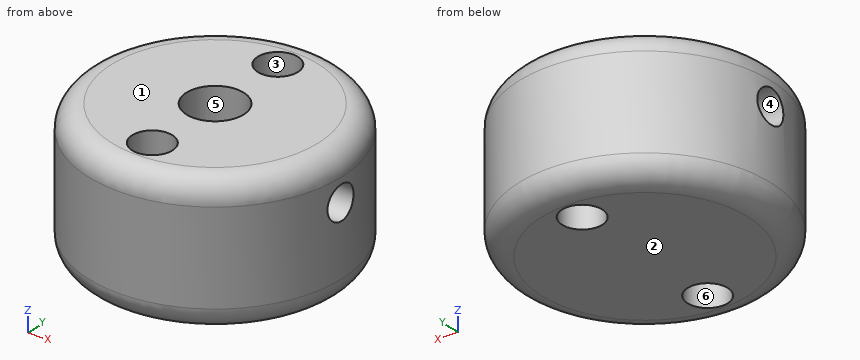
from build123d import *

# Parameters (mm, degrees)
SKETCH_1_R               = 11
EXTRUDE_1_DEPTH          = 12
SKETCH_3_R               = 1.75
CUT_EXTRUDE_1_DEPTH      = 20.646882704
SKETCH_4_R               = 2.5
CUT_EXTRUDE_2_DEPTH      = 10
CUT_EXTRUDE_3_DEPTH      = 20.646882704
CUT_EXTRUDE_3_DEPTH_BACK = 20.646882704
SKETCH_5_R               = 1.45
FILLET_1_R               = 2


with BuildPart() as part:
    # 草图1 → 凸台-拉伸1 (new body)
    with BuildSketch(Plane.XY):
        Circle(SKETCH_1_R)
    extrude(amount=EXTRUDE_1_DEPTH)

    # 草图3 → 切除-拉伸1 (cut, through all)
    with BuildSketch(Plane.XY.offset(12)):
        with Locations((0, 7)):
            Circle(SKETCH_3_R)
        with Locations((0, -7)):
            Circle(SKETCH_3_R)
    extrude(amount=-CUT_EXTRUDE_1_DEPTH, mode=Mode.SUBTRACT)

    # 草图4 → 切除-拉伸2 (cut)
    with BuildSketch(Plane.XY.offset(12)):
        Circle(SKETCH_4_R)
    extrude(amount=-CUT_EXTRUDE_2_DEPTH, mode=Mode.SUBTRACT)

    # 草图5 → 切除-拉伸3 (cut, two sides: drawn at the far end of the back side and taken through both)
    with BuildSketch(Plane(origin=(0, 0, 0), x_dir=(0, 0, -1), z_dir=(1, 0, 0)).offset(-CUT_EXTRUDE_3_DEPTH_BACK)):
        with Locations((-8, 0)):
            Circle(SKETCH_5_R)
    extrude(amount=CUT_EXTRUDE_3_DEPTH + CUT_EXTRUDE_3_DEPTH_BACK, mode=Mode.SUBTRACT)

    # 圆角1
    fillet_1_edges = [part.edges().sort_by_distance(p)[0] for p in [
        (-11, 0, 0),
        (-11, 0, 12),
    ]]
    fillet(fillet_1_edges, radius=FILLET_1_R)


solid = part.part
The listing builds one solid part. Answer for the finished solid, in the listing's coordinates (mm). Face numbers are marked on the shaded views. A direction names the side the tool comes from. Round coordinates to 2 decimals unless told otherwise and drop trailing zeros. Write each loop counter-clockwise with the first axis right and the second up, starting at its lowest first coordinate (ties: lowest second). Pieces come first, ordered by that corner, then holes. Notation, with made-up numbers: M 25.5,-19 L 62.5,-19 A16 cw 62.5,11 Z; hole C 69,-22.5 d3. An arc over 180 degrees is marked long. Write each question's results on one line, items separated by ' | '. Start each with the question number.
Item 1: A cutting plane is placed at A-A on z = 8. Write down the section's boundary in (x, y), and give its area (3 significant figures).
Item 2: Flat-ended cylindrical pins translate along their axes: pin 1 Ø1.5 at (x, y) = (1, 1) entering from +Z; pin 2 Ø3 at (x, z) = (4.5, 6) entering from +Y; pin 3 Ø1.5 at (x, z) = (5.5, 4.5) entering from -Y. Find the tip coordinate at first contact, or state that the pin passes through.
Item 3: A cutting plane is placed at B-B on x = 0. Write down the section's boundary in (y, z), and give its area (3 significant figures).
Item 4: For the marked faces 5 and 6, determine the directions among +Z, -Z, +X, -X, +Y, -Y from which every point of the face is accessible in a straight line to the end or side of a thin tool.
Item 5: Straight lines are drawn through the part: L1, parallel to Y at x = 0, z = 9; L2, parallel to Z at x = 5.25, y = 0; L3, parallel to X at y = 0, z = 9.75. For each, find the intervals that lie inside material, in ascending order. Write a range as [from, to].
Item 6: A cutting plane is placed at D-D on z = 3.25. Write down the section's boundary in (x, y), and give its area (3 significant figures).
Item 7: For a pull along Z with two mould halves and no side action, classify the marked faces 1, 2, 3 and 4 as pulls with the +Z half, pulls with the -Z half, needs draft (parallel to the pull), parting line crosses it, or undercut.
Item 8: A cutting plane is placed at C-C on y = 0. Write down the section's boundary in (x, z), and give its area (3 significant figures).
Check sheet entries:
1) outline: M -10.9,-1.45 A11 ccw 10.9,-1.45 L 2.04,-1.45 A2.5 cw -2.04,-1.45 Z; M -10.9,1.45 L -2.04,1.45 A2.5 cw 2.04,1.45 L 10.9,1.45 A11 ccw Z; hole C 0,-7 d3.5; hole C 0,7 d3.5 | area: 291 mm²
2) pin 1: z = 2 | pin 2: y = 10.58 | pin 3: y = -9.92
3) outline: M -11,2 A2 ccw -9,0 L -8.75,0 L -8.75,12 L -9,12 A2 ccw -11,10 Z; M -5.25,0 L 5.25,0 L 5.25,12 L 2.5,12 L 2.5,2 L -2.5,2 L -2.5,12 L -5.25,12 Z; M 8.75,0 L 9,0 A2 ccw 11,2 L 11,10 A2 ccw 9,12 L 8.75,12 Z | area: 127 mm²
4) face 5: +Z | face 6: +Z, -Z
5) L1: [-11, -8.75], [-5.25, -2.5], [2.5, 5.25], [8.75, 11] | L2: [0, 6.55], [9.45, 12] | L3: [-11, -2.5], [2.5, 11]
6) outline: C 0,0 d22; hole C 0,0 d5; hole C 0,-7 d3.5; hole C 0,7 d3.5 | area: 341 mm²
7) face 1: pulls with the +Z half | face 2: pulls with the -Z half | face 3: needs draft | face 4: undercut
8) outline: M -11,2 A2 ccw -9,0 L 9,0 A2 ccw 11,2 L 11,6.55 L 2.5,6.55 L 2.5,2 L -2.5,2 L -2.5,6.55 L -11,6.55 Z; M -11,9.45 L -2.5,9.45 L -2.5,12 L -9,12 A2 ccw -11,10 Z; M 2.5,9.45 L 11,9.45 L 11,10 A2 ccw 9,12 L 2.5,12 Z | area: 161 mm²
